```python
from build123d import *

# Parameters (mm, degrees)
SKETCH3_R          = 0.7
CUT_EXTRUDE1_DEPTH = 4
SKETCH2_R          = 0.7
CUT_EXTRUDE2_DEPTH = 4


with BuildPart() as part:
    # Sketch1 → Revolve1 (revolve)
    with BuildSketch(Plane.XY, mode=Mode.PRIVATE) as revolve1_sk:
        Polygon((35.4, 37.5), (35.98589676, 36.243540344), (36.78589676, 36.243540344), (37.37179352, 37.5), (37.77179352, 37.5), (38.352443595, 36.254791895), (39.152443595, 36.254791895), (39.73309367, 37.5), (40.13309367, 37.5), (40.13309367, 4), (70, 4), (70, 0), (0, 0), (0, 4), (29.86690633, 4), (29.86690633, 37.5), (30.26690633, 37.5), (30.847556405, 36.254791895), (31.647556405, 36.254791895), (32.22820648, 37.5), (32.62820648, 37.5), (33.21410324, 36.243540344), (34.01410324, 36.243540344), (34.6, 37.5), align=None)
    revolve(revolve1_sk.sketch.rotate(Axis((0, 0, 0), (1, 0, 0)), 90), axis=Axis((0, 0, 0), (1, 0, 0)))

    # Sketch3 → Cut-Extrude1 (cut)
    with BuildSketch(Plane(origin=(40.13309367, 0, 0), x_dir=(0, 0, -1), z_dir=(1, 0, 0))):
        with Locations((36.5, 0)):
            Circle(SKETCH3_R)
    extrude(amount=-CUT_EXTRUDE1_DEPTH, mode=Mode.SUBTRACT)

    # Sketch2 → Cut-Extrude2 (cut)
    with BuildSketch(Plane.ZY.offset(-29.86690633)):
        with Locations((36.5, 0)):
            Circle(SKETCH2_R)
    extrude(amount=-CUT_EXTRUDE2_DEPTH, mode=Mode.SUBTRACT)


solid = part.part
```
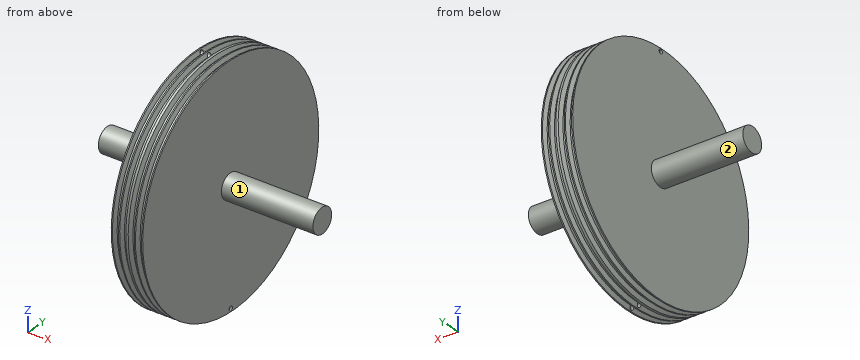
Input: part model. Units: mm. Frame: model coordinates. Face numbers are marked on the shaded views. A direction names the side the tool comes from. Coordinates: 2 decimals unless noted, no trailing zeros. Loops run counter-clockwise (first coordinate to the right, second up) from the corner with the lowest first, then second, coordinate; pieces in that order, holes last. Notation, with made-up numbers: M 53,62.5 L 74,62.5 A22 ccw 74,74.5 Z; hole C -20.5,44.5 d3. An arc over 180 degrees is marked long. One line per item, written item: value.
(1) Reachability of the marked faces 1 and 2 from +Z, -Z, +X, -X, +Y, -Y: full face, straight path, thin tool, end or side. Return the list, or none.
Filled in:
face 1: +X
face 2: -X
(2) Section A-A (x = 9). Output: boundary loops of the cut face in (y, z).
Filled in:
outline: C 0,0 d8
(3) Line query: line 1 along X through (y, z) = (-22.5, -15.5); line 2 along X through (y, z) = (19.5, 31.5); line 3 along Z through (x, y) = (46, -1). Output: solid intervals per line, ascending. Write a range as from..to.
Filled in:
line 1: 29.87..40.13
line 2: 29.87..30.48, 32.02..32.84, 34.39..35.61, 37.16..37.98, 39.52..40.13
line 3: -3.87..3.87
(4) Pin query (flat end, axial travel): pin 1 (4 mm diameter, centred on y = 8, z = -7, fed in from -X); pin 2 (1 mm diameter, centred on y = 20.5, z = 27, fed in from +X); pin 3 (3 mm diameter, centred on x = 26.5, z = 10.5, fed in from -Y); pin 4 (10 mm diameter, centred on x = 15.5, z = -0.5, fed in from +Y). Return the tip coordinate at first contact, or that it passes through.
Filled in:
pin 1: x = 29.87
pin 2: x = 40.13
pin 3: through
pin 4: y = 4
